from build123d import *

# Parameters (mm, degrees)
EXTRUDE_1_DEPTH          = 22
SKETCH_2_R               = 20
EXTRUDE_2_DEPTH          = 74
SKETCH_3_R               = 15
EXTRUDE_3_DEPTH          = 203
SKETCH_4_R               = 7.5
CUT_EXTRUDE_1_DEPTH      = 150
SKETCH_5_W               = 18
SKETCH_5_H               = 18
EXTRUDE_4_DEPTH          = 20
CUT_EXTRUDE_2_DEPTH      = 232.780607472
CUT_EXTRUDE_2_DEPTH_BACK = 232.780607472
CUT_EXTRUDE_3_DEPTH      = 232.780607472
CUT_EXTRUDE_3_DEPTH_BACK = 232.780607472
CHAMFER_1_SIZE           = 4
CHAMFER_2_SIZE           = 4
CUT_EXTRUDE_4_DEPTH      = 232.780607472
CUT_EXTRUDE_4_DEPTH_BACK = 232.780607472
SKETCH_8_R               = 3.25


with BuildPart() as part:
    # 草图1 → 凸台-拉伸1 (new body)
    with BuildSketch(Plane(origin=(0, 0, 0), x_dir=(1, 0, 0), z_dir=(0, 1, 0))):
        with BuildLine():
            Line((-20, -27.5), (20, -27.5))
            Line((20, -27.5), (20, 27.5))
            ThreePointArc((20, 27.5), (0, 47.5), (-20, 27.5))
            Line((-20, 27.5), (-20, -27.5))
        make_face()
    extrude(amount=EXTRUDE_1_DEPTH)

    # 草图2 → 凸台-拉伸2 (add)
    with BuildSketch(Plane(origin=(0, 22, 0), x_dir=(1, 0, 0), z_dir=(0, 1, 0))):
        with Locations(Location((0, 27.5, 0), (0, 0, 180))):
            Circle(SKETCH_2_R)
    extrude(amount=EXTRUDE_2_DEPTH)

    # 草图3 → 凸台-拉伸3 (add)
    with BuildSketch(Plane(origin=(0, 22, 0), x_dir=(1, 0, 0), z_dir=(0, 1, 0))):
        with Locations(Location((0, -8.5, 0), (0, 0, 90))):
            Circle(SKETCH_3_R)
    extrude(amount=EXTRUDE_3_DEPTH)

    # 草图4 → 切除-拉伸1 (cut)
    with BuildSketch(Plane(origin=(0, 225, 0), x_dir=(1, 0, 0), z_dir=(0, 1, 0))):
        with Locations(Location((0, -8.5, 0), (0, 0, 270))):
            Circle(SKETCH_4_R)
    extrude(amount=-CUT_EXTRUDE_1_DEPTH, mode=Mode.SUBTRACT)

    # 草图5 → 凸台-拉伸4 (add)
    with BuildSketch(Plane.XZ):
        with Locations((0, 8.5)):
            Rectangle(SKETCH_5_W, SKETCH_5_H)
    extrude(amount=EXTRUDE_4_DEPTH)

    # 草图6 → 切除-拉伸2 (cut, two sides: drawn at the far end of the back side and taken through both)
    with BuildSketch(Plane.ZY.offset(9).offset(-CUT_EXTRUDE_2_DEPTH_BACK)):
        with BuildLine():
            Line((8.5, -20), (-0.5, -20))
            Line((-0.5, -20), (-0.5, -11))
            ThreePointArc((-0.5, -11), (2.136038969, -17.363961031), (8.5, -20))
        make_face()
    extrude(amount=CUT_EXTRUDE_2_DEPTH + CUT_EXTRUDE_2_DEPTH_BACK, mode=Mode.SUBTRACT)

    # 草图7 → 切除-拉伸3 (cut, two sides: drawn at the far end of the back side and taken through both)
    with BuildSketch(Plane.ZY.offset(9).offset(-CUT_EXTRUDE_3_DEPTH_BACK)):
        with BuildLine():
            Line((8.5, -20), (17.5, -20))
            Line((17.5, -20), (17.5, -11))
            ThreePointArc((17.5, -11), (14.863961031, -17.363961031), (8.5, -20))
        make_face()
    extrude(amount=CUT_EXTRUDE_3_DEPTH + CUT_EXTRUDE_3_DEPTH_BACK, mode=Mode.SUBTRACT)

    # 倒角1
    chamfer_1_edges = [part.edges().sort_by_distance(p)[0] for p in [
        (-9, -5.5, -0.5),
        (-9, -20, 8.5),
        (-9, -5.5, 17.5),
    ]]
    chamfer(chamfer_1_edges, length=CHAMFER_1_SIZE)

    # 倒角2
    chamfer_2_edges = [part.edges().sort_by_distance(p)[0] for p in [
        (9, -5.5, -0.5),
        (9, -20, 8.5),
        (9, -5.5, 17.5),
    ]]
    chamfer(chamfer_2_edges, length=CHAMFER_2_SIZE)

    # 草图8 → 切除-拉伸4 (cut, two sides: drawn at the far end of the back side and taken through both)
    with BuildSketch(Plane(origin=(9, 0, 0), x_dir=(0, 0, -1), z_dir=(1, 0, 0)).offset(-CUT_EXTRUDE_4_DEPTH_BACK)):
        with Locations((-8.5, -10)):
            Circle(SKETCH_8_R)
    extrude(amount=CUT_EXTRUDE_4_DEPTH + CUT_EXTRUDE_4_DEPTH_BACK, mode=Mode.SUBTRACT)


solid = part.part
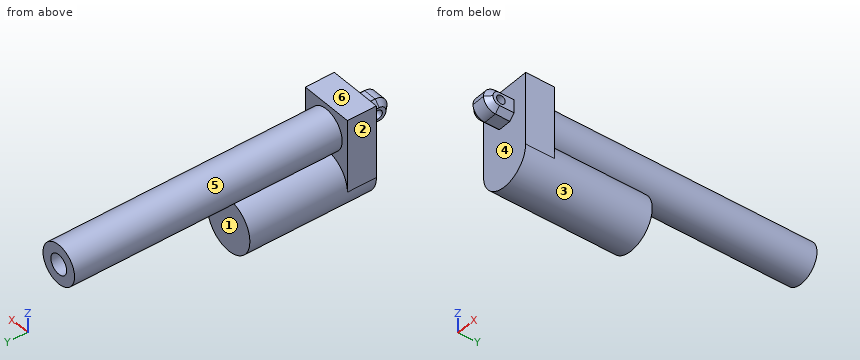
The model under review builds one solid part; all positions refer to its coordinate system, in mm. Face numbers are marked on the shaded views. A direction names the side the tool comes from. Give positions to 0.01 mm unless a question says otherwise; leave off trailing zeros. Loops run counter-clockwise (first coordinate to the right, second up) from the corner with the lowest first, then second, coordinate; pieces in that order, holes last. Notation, with made-up numbers: (49.5, 31) -> (97.5, 31) arc R14 ccw to (97.5, 38) -> close; hole circle Ø11 at (80.25, -15). An arc over 180 degrees is marked (long way). Write each question's results on one line, items separated by ' | '.
1) Insertion check: pin 1 Ø6 at (x, z) = (13.5, -26.5) entering from -Y; pin 2 Ø9 at (x, z) = (0, 8.5) entering from +Y; pin 3 Ø2 at (x, z) = (-12, -14) entering from +Y; pin 4 Ø6 at (y, z) = (-10, 8.5) entering from -X (3 decimals). Each pin has a flat end and moves straight along its axis. Give the tip position at first contact, or say it passes through.
Conclusion:
pin 1: stops at y = 0 | pin 2: stops at y = 75 | pin 3: stops at y = 96 | pin 4: passes through
2) Take a section at A-A, the plane z = -11.5. Give the boundary of the cut face in (x, y), plus the area to 3 significant figures.
Conclusion:
outline: (-20, 0) -> (20, 0) -> (20, 22) -> (12, 22) -> (12, 96) -> (-12, 96) -> (-12, 22) -> (-20, 22) -> close | area: 2,660 mm^2
3) Tool access review of the marked faces 1, 2 and 3: name each direction out of +Z, -Z, +X, -X, +Y, -Y from which nothing blocks a thin tool from reaching the whole face with its end or side.
Conclusion:
face 1: -Z, +X, -X, +Y | face 2: +Z, -Z, -X, +Y, -Y | face 3: +Y
4) Take a section at B-B, the plane y = 6. Give the boundary of the cut face in (x, z).
Conclusion:
outline: (-20, -27.5) arc R20 ccw to (20, -27.5) -> (20, 27.5) -> (-20, 27.5) -> close
5) For line 1 along X through (y, z) = (129.5, 8.5); line 2 along Z through (x, y) = (2.75, -10); line 3 along Z through (x, y) = (-0.5, 138), list the stretches that pass through material, from the lowest coordinate up. Write a range as from..to.
Conclusion:
line 1: x = -15..-7.5, 7.5..15 | line 2: z = -0.5..5.25, 11.75..17.5 | line 3: z = -6.49..1.02, 15.98..23.49
6) Draft analysis for pull direction Z (two halves, no side actions). For the marked faces 4, 5 and 6, state which applies: pulls with the +Z half, pulls with the -Z half, needs draft (parallel to the pull), parting line crosses it, or undercut.
Conclusion:
face 4: needs draft | face 5: undercut | face 6: pulls with the +Z half
